Could you check a few things on this model? Use its own coordinates, in mm. Face numbers are marked on the shaded views. A direction names the side the tool comes from. Give positions to 0.01 mm unless a question says otherwise; leave off trailing zeros. Loops run counter-clockwise (first coordinate to the right, second up) from the corner with the lowest first, then second, coordinate; pieces in that order, holes last. Notation, with made-up numbers: (-26.75, -0.75) - (-12.75, -0.75) arc R21 cw to (-12.75, 26.25) - close; hole circle Ø3 at (39, -17.75). An arc over 180 degrees is marked (long way). One line per item, written item: value. Start each with the question number.
Q1. For the marked faces 1, 2 and 3, which set-ups out of +Z, -Z, +X, -X, +Y, -Y let a thin tool reach every point of the face, with its end or its side?
Q2. I'm going to push flat-ended pins straight in: P1, Ø3.5, axis at y = 8, z = 4.5, coming from the -X side; P2, Ø5, axis at x = 3.52, y = 17, coming from the +Z side; P3, Ø3, axis at x = 20, z = 2, coming from the +Y side; P4, Ø2, axis at y = 24, z = 6.5, coming from the +X side. Where does each tip first touch, or does it pass through?
Q3. I want a section at C-C (y = 17.5). Please give me the cut outline in (x, z).
Q4. I want a section at B-B (x = 16.5). Please give me the cut outline in (y, z).
Q5. If we mould it in two halves opening along Y, with no side actions, what happens to the marked faces 4, 5 and 6? For each: released by +Y, released by -Y, zero draft, split by the parting line, or undercut.
Q6. I want a section at D-D (z = 0.75). Please give me the cut outline in (x, y), then the cut area to 3 significant figures.
Q7. I want a section at A-A (z = 4.25). Please give me the cut outline in (x, y).
Q8. If I drill on line 1 (Y direction, x = -12, z = 12.5); line 2 (X direction, y = 9.5, z = 3.25); line 3 (Y direction, x = 2, z = 1.5), over which ranges is the centre line in solid material (lowest first)? Write a range as from..to.
```python
from build123d import *

# Parameters (mm, degrees)
SKETCH_1_W          = 40
SKETCH_1_H          = 20
EXTRUDE_1_DEPTH     = 5
SKETCH_2_R          = 4
EXTRUDE_2_DEPTH     = 20
SKETCH_3_R          = 2.75
CUT_EXTRUDE_1_DEPTH = 36.595319622


with BuildPart() as part:
    # 草图1 → 凸台-拉伸1 (new body)
    with BuildSketch(Plane(origin=(0, 0, 0), x_dir=(1, 0, 0), z_dir=(0, 1, 0))):
        with Locations((3.522012579, -5.157232704)):
            Rectangle(SKETCH_1_W, SKETCH_1_H)
    extrude(amount=EXTRUDE_1_DEPTH)

    # 草图2 → 凸台-拉伸2 (add)
    with BuildSketch(Plane.XY.offset(15.157232704)):
        with BuildLine():
            Line((-6.477987421, 17), (-6.477987421, 5))
            Line((-6.477987421, 5), (13.522012579, 5))
            Line((13.522012579, 5), (13.522012579, 17))
            ThreePointArc((13.522012579, 17), (3.522012579, 27), (-6.477987421, 17))
        make_face()
        with Locations((3.522012579, 17)):
            Circle(SKETCH_2_R, mode=Mode.SUBTRACT)
    extrude(amount=-EXTRUDE_2_DEPTH)

    # 草图3 → 切除-拉伸1 (cut, through all)
    with BuildSketch(Plane(origin=(0, 5, 0), x_dir=(1, 0, 0), z_dir=(0, 1, 0))):
        with Locations(Location((-11.477987421, -5.157232704, 0), (0, 0, 270))):
            Circle(SKETCH_3_R)
        with Locations(Location((18.522012579, -5.157232704, 0), (0, 0, 270))):
            Circle(SKETCH_3_R)
    extrude(amount=-CUT_EXTRUDE_1_DEPTH, mode=Mode.SUBTRACT)


solid = part.part
```
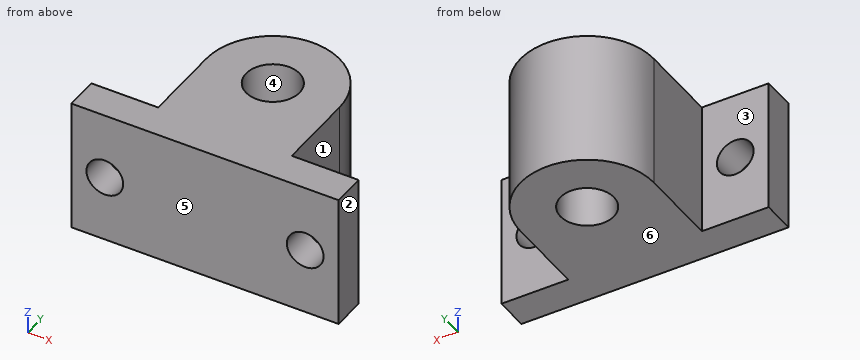
Worked answers:
1. face 1: +Z, -Z, +X, +Y
1. face 2: +Z, -Z, +X, +Y, -Y
1. face 3: +Z, -Z, -X, +Y
2. P1: stops at x = -6.48
2. P2: passes through
2. P3: stops at y = 5
2. P4: stops at x = 11.52
3. outline: (-6.47, -4.84) - (-0.45, -4.84) - (-0.45, 15.16) - (-6.47, 15.16) - close; (7.49, -4.84) - (13.51, -4.84) - (13.51, 15.16) - (7.49, 15.16) - close
4. outline: (0, -4.84) - (5, -4.84) - (5, 3.29) - (0, 3.29) - close; (0, 7.02) - (5, 7.02) - (5, 15.16) - (0, 15.16) - close
5. face 4: undercut
5. face 5: released by -Y
5. face 6: zero draft
6. outline: (-16.48, 0) - (23.52, 0) - (23.52, 5) - (13.52, 5) - (13.52, 17) arc R10 ccw to (-6.48, 17) - (-6.48, 5) - (-16.48, 5) - close; hole circle Ø8 at (3.52, 17)
6. area: 547 mm²
7. outline: (-16.48, 0) - (-14.07, 0) - (-14.07, 5) - (-16.48, 5) - close; (-8.88, 0) - (15.93, 0) - (15.93, 5) - (13.52, 5) - (13.52, 17) arc R10 ccw to (-6.48, 17) - (-6.48, 5) - (-8.88, 5) - close; (21.12, 0) - (23.52, 0) - (23.52, 5) - (21.12, 5) - close; hole circle Ø8 at (3.52, 17)
8. line 1: y = 0..5
8. line 2: x = -6.48..13.52
8. line 3: y = 0..13.3, 20.7..26.88
